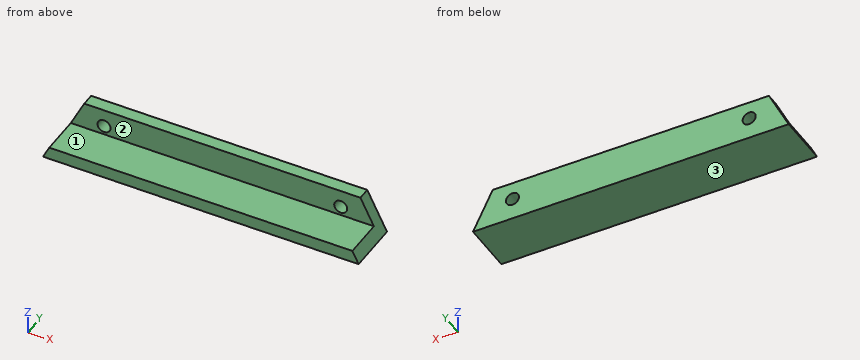
```python
from build123d import *

# Parameters (mm, degrees)
SKETCH1_R           = 1.65
BOSS_EXTRUDE1_DEPTH = 3.175
BOSS_EXTRUDE2_DEPTH = 10


with BuildPart() as part:
    # Sketch1 → Boss-Extrude1 (new body)
    with BuildSketch(Plane(origin=(0, 0, 0), x_dir=(1, 0, 0), z_dir=(0, 1, 0))):
        Polygon((-21.997084548, 0), (58.002915452, 0), (53.002915452, -10), (-16.997084548, -10), align=None)
        with Locations(Location((-11.997084548, -5.5, 0), (0, 0, 270))):
            Circle(SKETCH1_R, mode=Mode.SUBTRACT)
        with Locations(Location((48.002915452, -5.5, 0), (0, 0, 90))):
            Circle(SKETCH1_R, mode=Mode.SUBTRACT)
    extrude(amount=BOSS_EXTRUDE1_DEPTH)

    # Sketch2 → Boss-Extrude2 (add)
    with BuildSketch(Plane.XZ):
        Polygon((58.002915452, 0), (56.415415452, 3.175), (-20.409584548, 3.175), (-21.997084548, 0), align=None)
    extrude(amount=BOSS_EXTRUDE2_DEPTH)


solid = part.part
```
Source: CAD feature listing. Evaluate the final solid. Frame: model axes, mm. Face numbers are marked on the shaded views. Round coordinates to 2 decimals unless told otherwise and drop trailing zeros. Loops run counter-clockwise (first coordinate to the right, second up) from the corner with the lowest first, then second, coordinate; pieces in that order, holes last. Notation, with made-up numbers: M -28.75,66.5 L -20.75,66.5 A7 ccw -20.75,75.5 Z; hole C -39.75,-12 d6. An arc over 180 degrees is marked long. Use a Markdown table: item, result. Add a question column.
1. Section query C-C on y = -7.75. Return the cut outline in (x, z) (3 decimals), then the cut area to 3 significant figures.
2. Section query D-D on y = 1. Return the cut outline in (x, z).
3. Contact query for flat-ended pins moving along their axis: P1, Ø1, axis at x = 27, z = 6.5, coming from the -Y side; P2, Ø2, axis at x = 38, y = -5, coming from the +Z side (3 decimals); P3, Ø4, axis at y = -8.5, z = 5, coming from the +X side. Output: stop coordinate, or through.
4. Mould query, pull axis Z, two halves, no side actions, for the marked faces 1, 2 and 3. Classes: pulls with the +Z half, pulls with the -Z half, needs draft (parallel to the pull), parting line crosses it, or undercut.
5. Section query A-A on z = 5.5. Return the cut outline in (x, y) (3 decimals), then the cut area to 3 significant figures.
6. Section query B-B on x = 15.5. Return the cut outline in (y, z) (3 decimals).
7. Line query: line 1 (Z direction, x = 43, y = -3.5) (3 decimals); line 2 (X direction, y = 1.95, z = 5.5). Output: solid intervals per line, ascending.
Reported:
| question | item | result |
|---|---|---|
| 1 | outline | M -21.997,0 L 58.003,0 L 56.415,3.175 L -20.41,3.175 Z |
| 1 | area | 249 mm² |
| 2 | outline | M -22,0 L 58,0 L 53,10 L -17,10 Z; hole C -12,5.5 d3.3; hole C 48,5.5 d3.3 |
| 3 | P1 | stops at y = 0 |
| 3 | P2 | stops at z = 3.175 |
| 3 | P3 | stops at x = 56.5 |
| 4 | face 1 | pulls with the +Z half |
| 4 | face 2 | needs draft |
| 4 | face 3 | pulls with the -Z half |
| 5 | outline | M -19.247,0 L -13.647,0 L -13.647,3.175 L -19.247,3.175 Z; M -10.347,0 L 46.353,0 L 46.353,3.175 L -10.347,3.175 Z; M 49.653,0 L 55.253,0 L 55.253,3.175 L 49.653,3.175 Z |
| 5 | area | 216 mm² |
| 6 | outline | M -10,0 L 3.175,0 L 3.175,10 L 0,10 L 0,3.175 L -10,3.175 Z |
| 7 | line 1 | z = 0 to 3.175 |
| 7 | line 2 | x = -19.25 to -13.65, -10.35 to 46.35, 49.65 to 55.25 |
